Autodesk Inventor part; units mm, degrees
ref_plane "YZ Plane" through (0, 0, 0) normal (1, 0, 0) x (0, 1, 0)
ref_plane "XZ Plane" through (0, 0, 0) normal (0, 1, 0) x (-1, 0, 0)
ref_plane "XY Plane" through (0, 0, 0) normal (0, 0, 1) x (1, 0, 0)
sketch "Skizze1" plane through (0, 0, 0) normal (0, 0, 1) x (1, 0, 0)
  circle A0 centre (0, 0) radius 7.5
  dimension "d0" = 15
extrude "Extrusion1" add sketch "Skizze1" along normal mid plane 400
sketch "Skizze3" plane through (0, 0, 0) normal (0, 1, 0) x (-1, 0, 0)
  circle A0 centre (0, 150) radius 2.5
  circle A1 centre (0, -150) radius 2.5
  point P0 (0, 0)
  dimension "d7" = 5
  dimension "d8" = 5
extrude "Extrusion3" cut sketch "Skizze3" along normal mid plane 15
properties part number "Stange test"
Can you work these out from the model? Positions are in its coordinate system, mm. Round coordinates to 2 decimals unless told otherwise and drop trailing zeros. Write each loop counter-clockwise with the first axis right and the second up, starting at its lowest first coordinate (ties: lowest second). Pieces come first, ordered by that corner, then holes. Notation, with made-up numbers: M 83.5,60 L 109.5,60 A20 cw 109.5,99 Z; hole C 3.5,42.25 d8. An arc over 180 degrees is marked long. Use a Markdown table: item, result.
Item 1: We'd pull the mould along Y, two halves only. Please class faces 1 (the face through (-7.493, -0.33, -2.8)), 2 (the face through (0, 0, -200)): released by +Y, released by -Y, zero draft, split by the parting line, or undercut.
Found:
| item | result |
|---|---|
| face 1 | split by the parting line |
| face 2 | zero draft |
Item 2: If I drill on line 1 along Z through (x, y) = (0, 1.5); line 2 along Z through (x, y) = (-2, -5); line 3 along Y through (x, z) = (-0.75, -31), over which ranges is the centre line in solid material (lowest first)? Write a range as [from, to].
Found:
| item | result |
|---|---|
| line 1 | z = [-200, -152.5], [-147.5, 147.5], [152.5, 200] |
| line 2 | z = [-200, -151.5], [-148.5, 148.5], [151.5, 200] |
| line 3 | y = [-7.46, 7.46] |
Item 3: I want a section at A-A (x = 0). List the corners of the cut face in (y, z) for me.
Found:
| item | result |
|---|---|
| outline | M -7.5,-200 L 7.5,-200 L 7.5,-152.5 L -7.5,-152.5 Z; M -7.5,-147.5 L 7.5,-147.5 L 7.5,147.5 L -7.5,147.5 Z; M -7.5,152.5 L 7.5,152.5 L 7.5,200 L -7.5,200 Z |
Item 4: I want a section at C-C (z = -158.5). List the corners of the cut face in (x, y) for me, and give its area (3 significant figures).
Found:
| item | result |
|---|---|
| outline | C 0,0 d15 |
| area | 177 mm2 |
Item 5: I want a section at B-B (y = -4.5). List the corners of the cut face in (x, z) for me.
Found:
| item | result |
|---|---|
| outline | M -6,-200 L 6,-200 L 6,200 L -6,200 Z; hole C 0,-150 d5; hole C 0,150 d5 |
Item 6: For pin 1 Ø4 at (y, z) = (-3.5, -122.5) entering from +X; pin 2 Ø1 at (x, z) = (2, -84) entering from -Y; pin 3 Ø1.5 at (x, z) = (5.5, -131.5) entering from +Y, each with a flat end and sliding along its axis, tell me the tip position at first contact or that it passes through.
Found:
| item | result |
|---|---|
| pin 1 | stops at x = 7.35 |
| pin 2 | stops at y = -7.35 |
| pin 3 | stops at y = 5.8 |
